Autodesk Inventor part; units mm, degrees
ref_plane "YZ Plane" through (0, 0, 0) normal (1, 0, 0) x (0, 1, 0)
ref_plane "XZ Plane" through (0, 0, 0) normal (0, 1, 0) x (-1, 0, 0)
ref_plane "XY Plane" through (0, 0, 0) normal (0, 0, 1) x (1, 0, 0)
sketch "Sketch1" plane through (0, 0, 0) normal (0, 0, 1) x (1, 0, 0)
  circle A0 centre (0, 0) radius 6
  circle A1 centre (0, 0) radius 7
  dimension "d0" = 12
  dimension "d1" = 14
extrude "Extrusion1" add sketch "Sketch1" against normal mid plane 143.6
chamfer "Chamfer1" distance 0.1 angle 45 4 edges at (-6, 0, 71.8) (-7, 0, 71.8) (-7, 0, -71.8) (-6, 0, -71.8)
sketch "Sketch2" plane through (0, 0, 71.8) normal (0, 0, 1) x (1, 0, 0)
  circle A0 centre (0, 0) radius 6.5
  circle A1 centre (0, 0) radius 6
  dimension "d7" = 13
  dimension "d8" = 12
extrude "Extrusion2" cut sketch "Sketch2" against normal blind 20
sketch "Sketch3" plane through (0, 0, -71.8) normal (0, 0, -1) x (-1, 0, 0)
  circle A0 centre (0, 0) radius 6.5
  dimension "d11" = 13
extrude "Extrusion3" cut sketch "Sketch3" against normal blind 20
properties part number "Joint0_Joint1_Bushing"
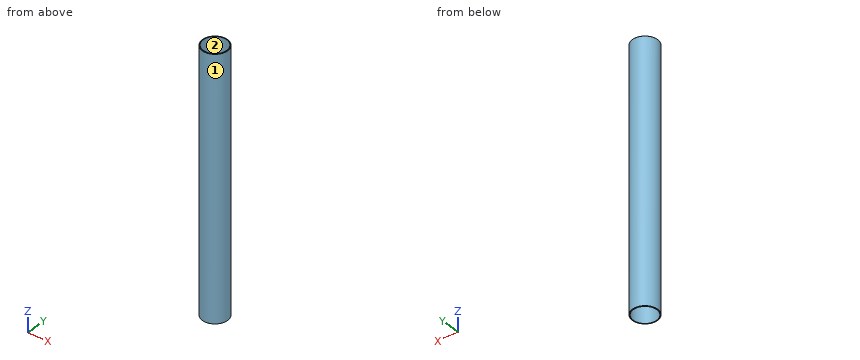
Work out the finished part from the listing and answer in its coordinate system (mm). Face numbers are marked on the shaded views. Round coordinates to 2 decimals unless told otherwise and drop trailing zeros. Write each loop counter-clockwise with the first axis right and the second up, starting at its lowest first coordinate (ties: lowest second). Pieces come first, ordered by that corner, then holes. Notation, with made-up numbers: (-27.5, 46.25) -> (17.5, 46.25) arc R22 ccw to (17.5, 58.25) -> close; hole circle Ø5 at (82, -25.5). An arc over 180 degrees is marked (long way). Write each question's results on one line, items separated by ' | '.
Item 1: A cutting plane is placed at A-A, the plane y = 0. Determine the outline of the cut face in (x, z).
Result set:
outline: (-7, -71.7) -> (-6.9, -71.8) -> (-6.5, -71.8) -> (-6.5, -51.8) -> (-6, -51.8) -> (-6, 51.8) -> (-6.5, 51.8) -> (-6.5, 71.8) -> (-6.9, 71.8) -> (-7, 71.7) -> close; (6, -51.8) -> (6.5, -51.8) -> (6.5, -71.8) -> (6.9, -71.8) -> (7, -71.7) -> (7, 71.7) -> (6.9, 71.8) -> (6.5, 71.8) -> (6.5, 51.8) -> (6, 51.8) -> close
Item 2: Find the intervals of material crossed by line 1 along Y through (x, z) = (0, -4.5); line 2 along Y through (x, z) = (0, 57); line 3 along X through (y, z) = (-1.25, 11.5), in increasing order. Write a range as [from, to].
Result set:
line 1: [-7, -6], [6, 7] | line 2: [-7, -6.5], [6.5, 7] | line 3: [-6.89, -5.87], [5.87, 6.89]
Item 3: A cutting plane is placed at D-D, the plane z = 57. Determine the outline of the cut face in (x, y).
Result set:
outline: circle Ø14 at (0, 0); hole circle Ø13 at (0, 0)
Item 4: Flat-ended cylindrical pins translate along their axes: P1, Ø1, axis at x = 5, y = -2.5, coming from the -Z side; P2, Ø1, axis at y = -2.5, z = -5.5, coming from the +X side; P3, Ø1, axis at x = -4, z = -47, coming from the +Y side. Find the tip coordinate at first contact, or state that the pin passes through.
Result set:
P1: z = -51.8 | P2: x = 6.71 | P3: y = 6.06
Item 5: The mould has two halves that part along X. Classify the marked faces 1 and 2: +X half, -X half, draft (parallel to the pull), parting line (faces both ways), or undercut.
Result set:
face 1: parting line | face 2: undercut
Item 6: A cutting plane is placed at C-C, the plane z = -31.5. Determine the outline of the cut face in (x, y), plus the area to 3 significant figures.
Result set:
outline: circle Ø14 at (0, 0); hole circle Ø12 at (0, 0) | area: 40.8 mm^2
